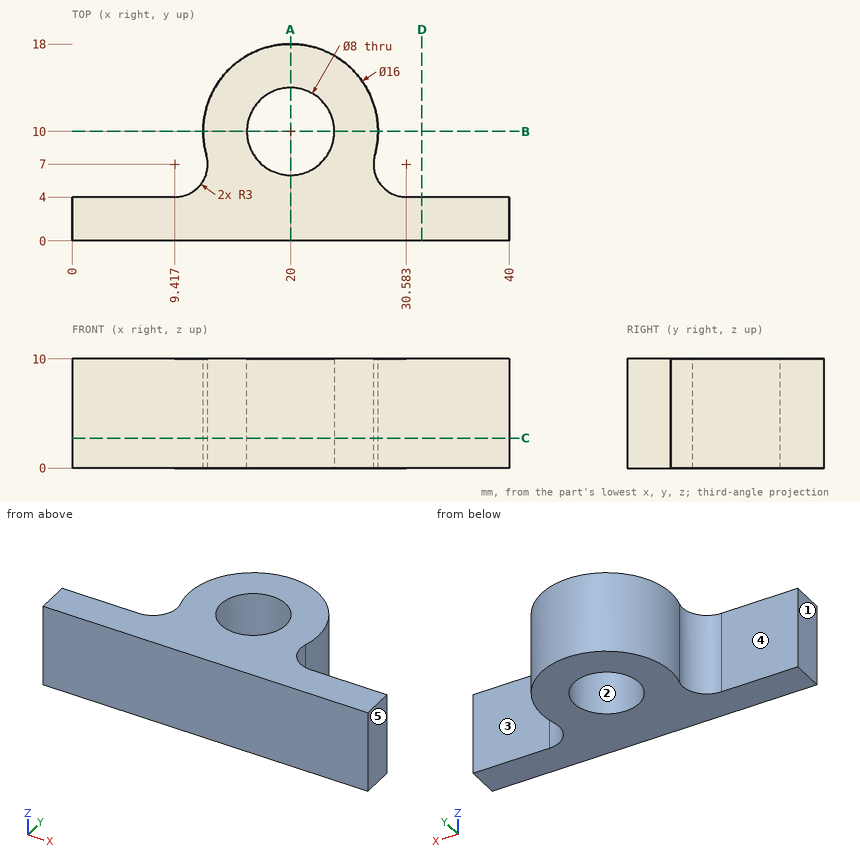
For this review, use the dimensioned drawing (mm, ordinates from the lowest corner) and the shaded views. A direction names the side the tool comes from. Give positions to 0.01 mm unless a question says otherwise; leave off trailing zeros. Loops run counter-clockwise (first coordinate to the right, second up) from the corner with the lowest first, then second, coordinate; pieces in that order, holes last. Notation, with made-up numbers: (-39, 68.5) -> (-11, 68.5) arc R22 cw to (-11, 99.5) -> close; hole circle Ø1 at (44, 2.25). An arc over 180 degrees is marked (long way). One line per question, with ' | ' between items. Start each with the question number.
(1) We need section C-C (z = 2.75). State the section outline as (x, y) points.
(2) Insertion check: P1, Ø1, axis at y = 8.5, z = 6, coming from the +X side; P2, Ø1, axis at x = 30, z = 8.5, coming from the +Y side. Each pin has a flat end and moves straight along its axis. Give the tip position at first contact, or say it passes through.
(3) For line 1 (Y direction, x = 20, z = 8); line 2 (X direction, y = 11, z = 2); line 3 (Y direction, x = 5.5, z = 4.75), list the stretches that pass through material, from the lowest coordinate up.
(4) We need section D-D (x = 32). State the section outline as (y, z) points.
(5) Draft analysis for pull direction X (two halves, no side actions). For the marked faces 1, 2 and 3, state which applies: +X half, -X half, draft (parallel to the pull), parting line (faces both ways), or undercut.
(6) We need section B-B (y = 10). State the section outline as (x, z) points, and give its area (3 significant figures).
(7) For the marked faces 4 and 5, list the 3-axis set-ups (+Z, -Z, +X, -X, +Y, -Y) from which the entire face can be reached by the end or side of a thin tool; tool diameter is ignored.
(8) We need section A-A (x = 20). State the section outline as (y, z) points, and give its area (3 significant figures).
The answers:
1) outline: (0, 0) -> (40, 0) -> (40, 4) -> (30.58, 4) arc R3 cw to (27.7, 7.82) arc R8 ccw (long way) to (12.3, 7.82) arc R3 cw to (9.42, 4) -> (0, 4) -> close; hole circle Ø8 at (20, 10)
2) P1: stops at x = 27.94 | P2: stops at y = 4.2
3) line 1: y = 0 to 6, 14 to 18 | line 2: x = 12.06 to 16.13, 23.87 to 27.94 | line 3: y = 0 to 4
4) outline: (0, 0) -> (4, 0) -> (4, 10) -> (0, 10) -> close
5) face 1: -X half | face 2: undercut | face 3: draft
6) outline: (12, 0) -> (16, 0) -> (16, 10) -> (12, 10) -> close; (24, 0) -> (28, 0) -> (28, 10) -> (24, 10) -> close | area: 80.0 mm^2
7) face 4: +Z, -Z, -X, +Y | face 5: +Z, -Z, +X, +Y, -Y
8) outline: (0, 0) -> (6, 0) -> (6, 10) -> (0, 10) -> close; (14, 0) -> (18, 0) -> (18, 10) -> (14, 10) -> close | area: 100 mm^2
